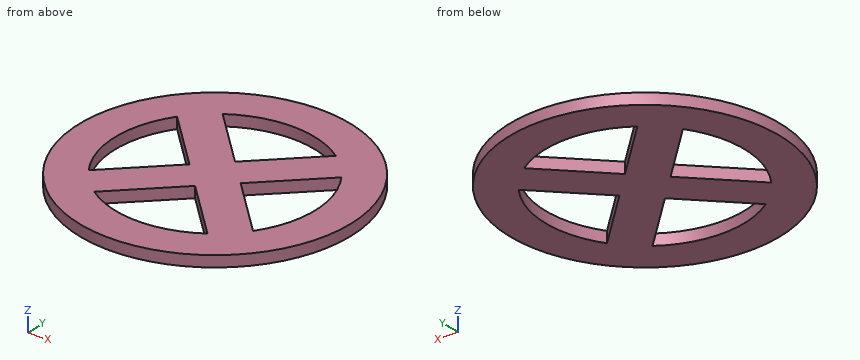
from build123d import *

# Parameters (mm, degrees)
F0_R     = 93.302436173
F1_DEPTH = 7.62


# Not quite as in the source:
# - ends of sketch curves that miss each other by under 0.0002 mm in the source are joined


with BuildPart() as f1:
    # F0 (on Top) → F1 (new body)
    with BuildSketch(Plane.XY):
        Circle(F0_R)
        with BuildLine():
            Line((-39.0521280378, -56.4777448198), (-0.032374081, -17.6012715653))
            Line((-0.032374081, -17.6012715653), (38.8440970553, -56.6210251423))
            ThreePointArc((38.8440970553, -56.6210251423), (-0.1262993869, -68.6643168805), (-39.0521280378, -56.4777448198))
        make_face(mode=Mode.SUBTRACT)
        with BuildLine():
            Line((56.477744538, -39.0521284453), (17.6012712801, -0.0323744851))
            Line((17.6012712801, -0.0323744851), (56.6210244822, 38.8440980175))
            ThreePointArc((56.6210244822, 38.8440980175), (68.6643168811, -0.1262990512), (56.477744538, -39.0521284453))
        make_face(mode=Mode.SUBTRACT)
        with BuildLine():
            ThreePointArc((-56.6210254, -38.8440966797), (-68.6643168783, 0.1263005725), (-56.4777437302, 39.0521296136))
            Line((-56.4777437302, 39.0521296136), (-17.6012714166, 0.0323766012))
            Line((-17.6012714166, 0.0323766012), (-56.6210254, -38.8440966797))
        make_face(mode=Mode.SUBTRACT)
        with BuildLine():
            Line((39.0521279012, 56.4777449142), (0.0323739658, 17.601271681))
            Line((0.0323739658, 17.601271681), (-38.8440980887, 56.6210244334))
            ThreePointArc((-38.8440980887, 56.6210244334), (0.1262986773, 68.6643168818), (39.0521279012, 56.4777449142))
        make_face(mode=Mode.SUBTRACT)
    extrude(amount=F1_DEPTH)


solid = f1.part
Work out the finished part from the listing and answer in its coordinate system (mm). Round coordinates to 2 decimals unless told otherwise and drop trailing zeros. Write each loop counter-clockwise with the first axis right and the second up, starting at its lowest first coordinate (ties: lowest second). Pieces come first, ordered by that corner, then holes.
1) Straight lines are drawn through the part: line 1 (Y direction, x = 1.5, z = 2.75); line 2 (X direction, y = 27.5, z = 4.5); line 3 (X direction, y = 29, z = 6.5). For each, find the intervals that lie inside material, in ascending order.
2) A cutting plane is placed at A-A (z = 3). Give the vertices of the cut face in (x, y), plus the area to 3 significant figures.
3) A cutting plane is placed at B-B (x = -14.5). Give the vertices of the cut face in (y, z), plus the area to 3 significant figures.
4) Given pin 1 Ø3 at (x, y) = (-10.5, 69.5) entering from -Z; pin 2 Ø1.5 at (x, z) = (-70.5, 4.5) entering from -Y; pin 3 Ø1 at (x, z) = (-54.5, 4.5) entering from +Y; pin 4 Ø1.5 at (y, z) = (-41, 3.5) entering from -X, each flat-ended and moving along its own axis, determine where each tip first touches the part or whether it passes through.
5) A cutting plane is placed at C-C (y = 61). Give the vertices of the cut face in (x, z), plus the area to 3 significant figures.
6) A cutting plane is placed at D-D (x = -48). Give the vertices of the cut face in (y, z).
Completed:
1. line 1: y = -93.29 to -68.65, -19.14 to 19.06, 68.65 to 93.29
1. line 2: x = -89.16 to -62.92, -44.97 to -9.83, 9.97 to 45.24, 62.92 to 89.16
1. line 3: x = -88.68 to -62.24, -46.46 to -11.32, 11.47 to 46.74, 62.24 to 88.68
2. outline: circle Ø186.6 at (0, 0); hole (-56.62, -38.84) - (-17.6, 0.03) - (-56.48, 39.05) arc R68.66 ccw to start; hole (-39.05, -56.48) arc R68.66 ccw to (38.84, -56.62) - (-0.03, -17.6) - close; hole (-38.84, 56.62) - (0.03, 17.6) - (39.05, 56.48) arc R68.66 ccw to start; hole (17.6, -0.03) - (56.48, -39.05) arc R68.66 ccw to (56.62, 38.84) - close
2. area: 18,700 mm2
3. outline: (-92.17, 0) - (-67.12, 0) - (-67.12, 7.62) - (-92.17, 7.62) - close; (-32.02, 0) - (32.19, 0) - (32.19, 7.62) - (-32.02, 7.62) - close; (67.12, 0) - (92.17, 0) - (92.17, 7.62) - (67.12, 7.62) - close
3. area: 871 mm2
4. pin 1: stops at z = 0
4. pin 2: stops at y = -61.97
4. pin 3: stops at y = 76.09
4. pin 4: stops at x = -84.17
5. outline: (-70.6, 0) - (-31.52, 0) - (-31.52, 7.62) - (-70.6, 7.62) - close; (31.52, 0) - (70.6, 0) - (70.6, 7.62) - (31.52, 7.62) - close
5. area: 596 mm2
6. outline: (-80.01, 0) - (-30.25, 0) - (-30.25, 7.62) - (-80.01, 7.62) - close; (30.54, 0) - (80.01, 0) - (80.01, 7.62) - (30.54, 7.62) - close
